Autodesk Inventor part; units mm, degrees
ref_plane "YZ Plane" through (0, 0, 0) normal (1, 0, 0) x (0, 1, 0)
ref_plane "XZ Plane" through (0, 0, 0) normal (0, 1, 0) x (-1, 0, 0)
ref_plane "XY Plane" through (0, 0, 0) normal (0, 0, 1) x (1, 0, 0)
sketch "Sketch1" plane through (0, 0, 0) normal (0, 1, 0) x (-1, 0, 0)
  line L0 (0, 0) -> (0, -31.748)
  line L1 (0, -31.748) -> (7.62, -31.748)
  line L2 (7.62, -31.748) -> (7.62, -26.16)
  line L3 (7.62, -26.16) -> (4.953, -26.16)
  line L4 (4.953, -26.16) -> (4.953, -23.493)
  line L5 (4.953, -23.493) -> (7.62, -23.493)
  line L6 (7.62, -23.493) -> (7.62, -17.016)
  line L7 (7.62, -17.016) -> (2.54, -17.016)
  line L8 (2.54, -17.016) -> (2.54, 0)
  line L9 (0, 0) -> (2.54, 0)
  dimension "d0" = 31.748
  dimension "d1" = 7.62
  dimension "d2" = 5.588
  dimension "d3" = 2.667
  dimension "d4" = 2.667
  dimension "d5" = 6.477
  dimension "d6" = 5.08
  dimension "d7" = 2.54
revolve "Revolution1" add sketch "Sketch1" angle 360 about axis through (0, 0, 0) along (-1, 0, 0)
sketch "Sketch2" plane through (-7.62, 0, 0) normal (-1, 0, 0) x (0, 0, 1)
  circle A0 centre (28.954, 0) radius 1.5
  circle A1 centre (0, 0) radius 31.748
  line L0 (31.748, 0) -> (26.16, 0)
  circle A2 centre (0, 0) radius 26.16
  circle A3 centre (0, 28.954) radius 1.5
  circle A4 centre (-28.954, 0) radius 1.5
  circle A5 centre (0, -28.954) radius 1.5
  dimension "d9" = 3
  dimension "d12" = 360
extrude "Extrusion1" cut sketch "Sketch2" against normal blind 12.7 contours L0 A0 | A0 L0 | A3 | A4 | A5
sketch "Sketch3" plane through (0, 0, 0) normal (1, 0, 0) x (0, 0, -1)
  circle A0 centre (0, 0) radius 23.493
  circle A1 centre (0, 0) radius 20.2545
  circle A2 centre (20.2545, 0) radius 1.5
  circle A3 centre (0, 20.2545) radius 1.5
  circle A4 centre (-20.2545, 0) radius 1.5
  circle A5 centre (0, -20.2545) radius 1.5
  dimension "d17" = 3.2385
  dimension "d18" = 3
  dimension "d21" = 360
sketch "Sketch4" plane through (-7.62, 0, 0) normal (-1, 0, 0) x (0, 0, 1)
  circle A0 centre (0, 0) radius 17.016
  circle A1 centre (0, 0) radius 23.493
  dimension "d16" = 6.477
extrude "Extrusion2" cut sketch "Sketch3" against normal blind 5.08 contours A1 A2 | A1 A2 | A3 A1 | A1 A3 | A5 A1 | A1 A5 | A4 A1 | A1 A4
sketch "Sketch5" plane through (-2.54, 0, 0) normal (-1, 0, 0) x (0, 0, 1)
  circle A0 centre (0, 0) radius 17.016
  line L0 (-17.016, 0) -> (17.016, 0)
  line L1 (-14.478, -9.9949) -> (14.478, -9.9949)
  line L2 (-14.478, 9.9949) -> (14.478, 9.9949)
  line L3 (14.478, 9.9949) -> (14.478, -9.9949)
  line L4 (-14.478, 9.9949) -> (-14.478, -9.9949)
  arc A1 (16.8267, -2.5309) -> (16.8267, 2.5309) centre (0, 0) ccw
  point P0 (0, 9.9949)
  point P1 (14.478, 0)
  dimension "d25" = 28.956
  dimension "d26" = 19.9898
sketch "Sketch6" plane through (-7.62, 0, 0) normal (-1, 0, 0) x (0, 0, 1)
  circle A0 centre (0, 0) radius 17.016
  circle A1 centre (17.016, 0) radius 2.54
  arc A2 (16.8264, -2.5329) -> (16.8264, 2.5329) centre (0, 0) ccw
  circle A3 centre (-17.016, -0.0173) radius 2.54
  arc A4 (-16.829, 2.5158) -> (-16.8238, -2.55) centre (0, 0) ccw
  dimension "d27" = 5.08
  dimension "d28" = 5.08
extrude "Extrusion3" cut sketch "Sketch6" against normal blind 12.7 contours A0 A1 | A3 A0 picked at (16.1885, -0.4913) picked at (-16.1553, -0.0173)
sketch "Sketch7" plane through (-2.54, 0, 17.016) normal (-1, 0, 0) x (0, 0, 1)
  arc A0 (-33.8398, -2.55) -> (-33.8449, 2.5158) centre (-34.0319, -0.0173) ccw
  line L0 (-31.4919, -0.0173) -> (-2.4894, -0.0173) construction
  line L1 (-25.6012, 5.588) -> (-8.4308, 5.588)
  point P0 (-17.016, 0)
  point P1 (-17.016, 5.588)
  dimension "d34" = 5.588
hole "Hole1" at (-2.54, 5.588, -8.5852) at (-2.54, 5.588, 8.5852) direction (1, 0, 0) diameter 3.6576 depth 1.27 tip angle 118
equation "\"d28\" = d27"
properties part number "LED holder 2"
Geometry: final body of the model. Coordinates: model frame, mm. A direction names the side the tool comes from. Round coordinates to 2 decimals unless told otherwise and drop trailing zeros. Order: outer loops, then holes, each group sorted by start corner. A loop starts at its lowest first (then second) coordinate and runs counter-clockwise, first axis right, second up. Notation, with made-up numbers: (1.5, 35) -> (23.5, 35) arc R24 ccw to (23.5, 64) -> close; hole circle Ø7 at (-33.5, 12.25). An arc over 180 degrees is marked (long way). Put each result on its own line as item: value. Start each with the question number.
Q1. Line query: probe 1 along Y at (x, z) = (-1.75, 0); probe 2 along Y at (x, z) = (-7, 12.5); probe 3 along Z at (x, y) = (-7, -2). Output: solid intervals per line, ascending.
Q2. Section B-B on x = -6. Return the cut outline in (y, z).
Q3. First-contact query: pin 1 (1.5 mm diameter, centred on x = -3, z = 8, fed in from +Y); pin 2 (1.8 mm diameter, centred on y = 0, z = 20.25, fed in from +X); pin 3 (3.5 mm diameter, centred on y = 0, z = -28.954, fed in from +X); pin 4 (17 mm diameter, centred on y = -1, z = 1, fed in from -X). Flat tips, straight axial feed; report the tip coordinate or a pass-through.
Q4. Pull-direction query (Y, two-part tool) for faces 4 (the cylindrical face through (-1.288, 0.018, -17.016)), 5 (the flat face through (-7.62, -12, 24)); classes: +Y half, -Y half, draft (parallel to the pull), parting line (faces both ways), or undercut.
Q5. Section C-C on y = -14.5. Return the cut outline in (x, z).
Q6. Reachability of faces 1 (the flat face through (-2.54, 0, 0)), 2 (the flat face through (-5.08, 20, 0)), 3 (the cylindrical face through (-3.86, 30.44, -0.2)) from +Z, -Z, +X, -X, +Y, -Y: full face, straight path, thin tool, end or side. Return the list, or none.
Q7. Section A-A on z = 0. Give the number of separate pieces and of enclosed holes in the cut face, and give its area (3 significant figures).
Q8. Section D-D on z = 22.5. Return the cut outline in (x, y), and give its area (3 significant figures).
Ans:
1. probe 1: y = -31.75 to -30.45, -27.45 to -21.75, -18.75 to 18.75, 21.75 to 27.45, 30.45 to 31.75
1. probe 2: y = -29.18 to -22.98, -19.89 to -11.55, 11.55 to 19.89, 22.98 to 29.18
1. probe 3: z = -31.68 to -26.08, -23.41 to -16.9, 16.9 to 23.41, 26.08 to 31.68
2. outline: circle Ø63.5 at (0, 0); circle Ø46.99 at (0, 0); hole circle Ø3 at (-28.95, 0); hole circle Ø52.32 at (0, 0); hole circle Ø34.03 at (0, 0); hole circle Ø3 at (0, -28.95); hole circle Ø3 at (0, 28.95); hole circle Ø3 at (28.95, 0)
3. pin 1: stops at y = 30.91
3. pin 2: stops at x = -5.08
3. pin 3: stops at x = 0
3. pin 4: stops at x = -2.54
4. face 4: undercut
4. face 5: draft
5. outline: (-7.62, -28.24) -> (0, -28.24) -> (0, 28.24) -> (-7.62, 28.24) -> (-7.62, 21.77) -> (-4.95, 21.77) -> (-4.95, 18.48) -> (-7.62, 18.48) -> (-7.62, 8.9) -> (-2.54, 8.9) -> (-2.54, -8.9) -> (-7.62, -8.9) -> (-7.62, -18.48) -> (-4.95, -18.48) -> (-4.95, -21.77) -> (-7.62, -21.77) -> close
6. face 1: -X
6. face 2: +X
6. face 3: +X, -X
7. separate pieces: 3
7. enclosed holes: 0
7. area: 221 mm2
8. outline: (-7.62, -22.4) -> (0, -22.4) -> (0, 22.4) -> (-7.62, 22.4) -> (-7.62, 13.35) -> (-4.95, 13.35) -> (-4.95, 6.76) -> (-7.62, 6.76) -> (-7.62, -6.76) -> (-4.95, -6.76) -> (-4.95, -13.35) -> (-7.62, -13.35) -> close
8. area: 306 mm2
